from build123d import *

# Parameters (mm, degrees)
BOSS_EXTRUDE1_DEPTH = 4.51
CUT_EXTRUDE1_DEPTH  = 4.2
SKETCH6_R           = 0.65
BOSS_EXTRUDE2_DEPTH = 4.2
SKETCH7_R           = 0.55
CUT_EXTRUDE2_DEPTH  = 4.6
SKETCH8_R           = 0.5
CUT_EXTRUDE3_DEPTH  = 3.5
SKETCH10_R          = 0.5
SKETCH10_R_2        = 0.985
SKETCH10_R_3        = 0.9
SKETCH10_R_4        = 1
SKETCH10_R_5        = 0.75
CUT_EXTRUDE4_DEPTH  = 10
SKETCH16_W          = 2.4
SKETCH16_H          = 3
SKETCH16_H_2        = 1.5
CUT_EXTRUDE5_DEPTH  = 0.6
SKETCH18_W          = 1.5
SKETCH18_H          = 2.4
CUT_EXTRUDE6_DEPTH  = 1
SKETCH21_W          = 2.4
SKETCH21_H          = 1.5
SKETCH21_W_2        = 1.5
SKETCH21_H_2        = 8.25
CUT_EXTRUDE7_DEPTH  = 0.6
SKETCH22_R          = 1.3
SKETCH22_R_2        = 0.9
BOSS_EXTRUDE3_DEPTH = 4.25
SKETCH23_R          = 5.9
SKETCH23_R_2        = 5.5
BOSS_EXTRUDE4_DEPTH = 4
SKETCH24_R          = 1.6
SKETCH24_R_2        = 1.2
SKETCH24_R_3        = 1.25
SKETCH24_R_4        = 0.5
BOSS_EXTRUDE5_DEPTH = 3.75
SKETCH26_R          = 0.75
BOSS_EXTRUDE6_DEPTH = 4.51
SKETCH27_R          = 0.675
BOSS_EXTRUDE7_DEPTH = 4.6
BOSS_EXTRUDE8_DEPTH = 1.25
SKETCH29_W          = 0.2
SKETCH29_H          = 13.4
CUT_EXTRUDE8_DEPTH  = 15


with BuildPart() as part:
    # Sketch4 → Boss-Extrude1 (new body)
    with BuildSketch(Plane.XY):
        with BuildLine():
            ThreePointArc((-13.711599695, 0.852101617), (-13.847357447, 0.940933533), (-13.9, 1.09439375))
            Line((-13.9, 1.09439375), (-13.9, 24.20560625))
            ThreePointArc((-13.9, 24.20560625), (-13.847357447, 24.359066467), (-13.711599695, 24.447898383))
            Line((-13.711599695, 24.447898383), (-10.481270444, 25.269168531))
            ThreePointArc((-10.481270444, 25.269168531), (-10.359031781, 25.292262196), (-10.234871665, 25.3))
            Line((-10.234871665, 25.3), (-3.665128335, 25.3))
            ThreePointArc((-3.665128335, 25.3), (-3.540968219, 25.292262196), (-3.418729556, 25.269168531))
            Line((-3.418729556, 25.269168531), (-0.188400305, 24.447898383))
            ThreePointArc((-0.188400305, 24.447898383), (-0.052642553, 24.359066467), (0, 24.20560625))
            Line((0, 24.20560625), (0, 1.09439375))
            ThreePointArc((0, 1.09439375), (-0.052642553, 0.940933533), (-0.188400305, 0.852101617))
            Line((-0.188400305, 0.852101617), (-3.418729556, 0.030831469))
            ThreePointArc((-3.418729556, 0.030831469), (-3.540968219, 0.007737804), (-3.665128335, 0))
            Line((-3.665128335, 0), (-10.234871665, 0))
            ThreePointArc((-10.234871665, 0), (-10.359031781, 0.007737804), (-10.481270444, 0.030831469))
            Line((-10.481270444, 0.030831469), (-13.711599695, 0.852101617))
        make_face()
    extrude(amount=BOSS_EXTRUDE1_DEPTH)

    # Sketch5 → Cut-Extrude1 (cut)
    with BuildSketch(Plane(origin=(0, 0, 0), x_dir=(-1, 0, 0), z_dir=(0, 0, -1))):
        with BuildLine():
            Line((13.3, 1.366545), (13.3, 23.933455))
            Line((13.3, 23.933455), (10.333431177, 24.687667412))
            ThreePointArc((10.333431177, 24.687667412), (10.284535712, 24.696904878), (10.234871665, 24.7))
            Line((10.234871665, 24.7), (3.665128335, 24.7))
            ThreePointArc((3.665128335, 24.7), (3.615464288, 24.696904878), (3.566568823, 24.687667412))
            Line((3.566568823, 24.687667412), (0.6, 23.933455))
            Line((0.6, 23.933455), (0.6, 1.366545))
            Line((0.6, 1.366545), (3.566568823, 0.612332588))
            ThreePointArc((3.566568823, 0.612332588), (3.615464288, 0.603095122), (3.665128335, 0.6))
            Line((3.665128335, 0.6), (10.234871665, 0.6))
            ThreePointArc((10.234871665, 0.6), (10.284535712, 0.603095122), (10.333431177, 0.612332588))
            Line((10.333431177, 0.612332588), (13.3, 1.366545))
        make_face()
    extrude(amount=-CUT_EXTRUDE1_DEPTH, mode=Mode.SUBTRACT)

    # Sketch6 → Boss-Extrude2 (add)
    with BuildSketch(Plane(origin=(0, 0, 4.2), x_dir=(-1, 0, 0), z_dir=(0, 0, -1))):
        with Locations((1.112347538, 1.766545)):
            Circle(SKETCH6_R)
        with Locations((1.112347538, 23.533455)):
            Circle(SKETCH6_R)
        with Locations((1.11, 12.75)):
            Circle(SKETCH6_R)
        with Locations((12.787652462, 23.533455)):
            Circle(SKETCH6_R)
        with Locations((12.787652462, 1.766545)):
            Circle(SKETCH6_R)
        with Locations((12.79, 12.75)):
            Circle(SKETCH6_R)
    extrude(amount=BOSS_EXTRUDE2_DEPTH)

    # Sketch7 → Cut-Extrude2 (cut)
    with BuildSketch(Plane(origin=(0, 0, 0), x_dir=(-1, 0, 0), z_dir=(0, 0, -1))):
        with Locations((1.112347538, 1.766545)):
            Circle(SKETCH7_R)
        with Locations((1.11, 12.75)):
            Circle(SKETCH7_R)
        with Locations((1.112347538, 23.533455)):
            Circle(SKETCH7_R)
        with Locations(Location((12.787652462, 1.766545, 0), (0, 0, 180))):
            Circle(SKETCH7_R)
        with Locations(Location((12.787652462, 23.533455, 0), (0, 0, 180))):
            Circle(SKETCH7_R)
        with Locations(Location((12.79, 12.75, 0), (0, 0, 180))):
            Circle(SKETCH7_R)
    extrude(amount=-CUT_EXTRUDE2_DEPTH, mode=Mode.SUBTRACT)

    # Sketch8 → Cut-Extrude3 (cut)
    with BuildSketch(Plane(origin=(0, 0, 4.2), x_dir=(-1, 0, 0), z_dir=(0, 0, -1))):
        with Locations(Location((6.95, 24.2, 0), (0, 0, 90))):
            Circle(SKETCH8_R)
    extrude(amount=-CUT_EXTRUDE3_DEPTH, mode=Mode.SUBTRACT)

    # Sketch10 → Cut-Extrude4 (cut)
    with BuildSketch(Plane.XY.offset(4.51)):
        with Locations((-7.95, 19.1)):
            Circle(SKETCH10_R)
        with Locations((-3.95, 18.3)):
            Circle(SKETCH10_R_2)
        with Locations((-6.95, 13.6)):
            Circle(SKETCH10_R_3)
        with Locations((-6.95, 6.6)):
            Circle(SKETCH10_R_4)
        with Locations((-11.3, 17.35)):
            Circle(SKETCH10_R_5)
    extrude(amount=-CUT_EXTRUDE4_DEPTH, mode=Mode.SUBTRACT)

    # Sketch16 → Cut-Extrude5 (cut)
    with BuildSketch(Plane(origin=(0, 0, 0), x_dir=(0, 0, -1), z_dir=(1, 0, 0))):
        with Locations((-1.2, 16.3)):
            Rectangle(SKETCH16_W, SKETCH16_H)
        with Locations((-1.2, 11.35)):
            Rectangle(SKETCH16_W, SKETCH16_H_2)
        with Locations((-1.2, 3.25)):
            Rectangle(SKETCH16_W, SKETCH16_H_2)
    extrude(amount=-CUT_EXTRUDE5_DEPTH, mode=Mode.SUBTRACT)

    # Sketch18 → Cut-Extrude6 (cut)
    with BuildSketch(Plane(origin=(0, 0, 0), x_dir=(-1, 0, 0), z_dir=(0, -1, 0))):
        with Locations((2.95, -1.2)):
            Rectangle(SKETCH18_W, SKETCH18_H)
        with Locations((11.15, -1.2)):
            Rectangle(SKETCH18_W, SKETCH18_H)
    extrude(amount=-CUT_EXTRUDE6_DEPTH, mode=Mode.SUBTRACT)

    # Sketch21 → Cut-Extrude7 (cut)
    with BuildSketch(Plane.ZY.offset(13.9)):
        with Locations((1.2, 3.25)):
            Rectangle(SKETCH21_W, SKETCH21_H)
        with Locations((1.2, 11.35)):
            Rectangle(SKETCH21_W, SKETCH21_H)
        with Locations((0.75, 18.175)):
            Rectangle(SKETCH21_W_2, SKETCH21_H_2)
    extrude(amount=-CUT_EXTRUDE7_DEPTH, mode=Mode.SUBTRACT)

    # Sketch22 → Boss-Extrude3 (add)
    with BuildSketch(Plane(origin=(0, 0, 4.2), x_dir=(-1, 0, 0), z_dir=(0, 0, -1))):
        with Locations((6.95, 13.6)):
            Circle(SKETCH22_R)
        with Locations(Location((6.95, 13.6, 0), (0, 0, 180))):
            Circle(SKETCH22_R_2, mode=Mode.SUBTRACT)
    extrude(amount=BOSS_EXTRUDE3_DEPTH)

    # Sketch23 → Boss-Extrude4 (add)
    with BuildSketch(Plane(origin=(0, 0, 4.2), x_dir=(-1, 0, 0), z_dir=(0, 0, -1))):
        with Locations((6.95, 6.6)):
            Circle(SKETCH23_R)
        with Locations((6.95, 6.6)):
            Circle(SKETCH23_R_2, mode=Mode.SUBTRACT)
    extrude(amount=BOSS_EXTRUDE4_DEPTH)

    # Sketch24 → Boss-Extrude5 (add)
    with BuildSketch(Plane(origin=(0, 0, 4.2), x_dir=(-1, 0, 0), z_dir=(0, 0, -1))):
        with Locations((3.95, 18.3)):
            Circle(SKETCH24_R)
        with Locations((3.95, 18.3)):
            Circle(SKETCH24_R_2, mode=Mode.SUBTRACT)
        with Locations((7.95, 19.1)):
            Circle(SKETCH24_R_3)
        with Locations(Location((7.95, 19.1, 0), (0, 0, 180))):
            Circle(SKETCH24_R_4, mode=Mode.SUBTRACT)
    extrude(amount=BOSS_EXTRUDE5_DEPTH)

    # Sketch26 → Boss-Extrude6 (add)
    with BuildSketch(Plane.XY.offset(4.51)):
        with Locations((-11.3, 17.35)):
            Circle(SKETCH26_R)
    extrude(amount=-BOSS_EXTRUDE6_DEPTH)

    # Sketch27 → Boss-Extrude7 (add)
    with BuildSketch(Plane(origin=(0, 0, 0), x_dir=(-1, 0, 0), z_dir=(0, 0, -1))):
        with Locations((11.3, 17.35)):
            Circle(SKETCH27_R)
    extrude(amount=BOSS_EXTRUDE7_DEPTH)

    # Sketch28 → Boss-Extrude8 (add)
    with BuildSketch(Plane(origin=(0, 0, 0.45), x_dir=(-1, 0, 0), z_dir=(0, 0, -1))):
        with BuildLine():
            ThreePointArc((7.737135239, 20.331742097), (9.19542716, 19.206823169), (7.95, 17.85))
            ThreePointArc((7.95, 17.85), (7.865931561, 17.934068439), (7.95, 18.018136879))
            ThreePointArc((7.95, 18.018136879), (9.02656312, 19.206956355), (7.737135239, 20.160715045))
            ThreePointArc((7.737135239, 20.160715045), (7.728639485, 20.246228571), (7.737135239, 20.331742097))
        make_face()
    extrude(amount=BOSS_EXTRUDE8_DEPTH)

    # Sketch29 → Cut-Extrude8 (cut)
    with BuildSketch(Plane(origin=(0, 0, 0), x_dir=(0, 0, -1), z_dir=(1, 0, 0))):
        with Locations((-0.1, 6.7)):
            Rectangle(SKETCH29_W, SKETCH29_H)
    extrude(amount=-CUT_EXTRUDE8_DEPTH, mode=Mode.SUBTRACT)


solid = part.part
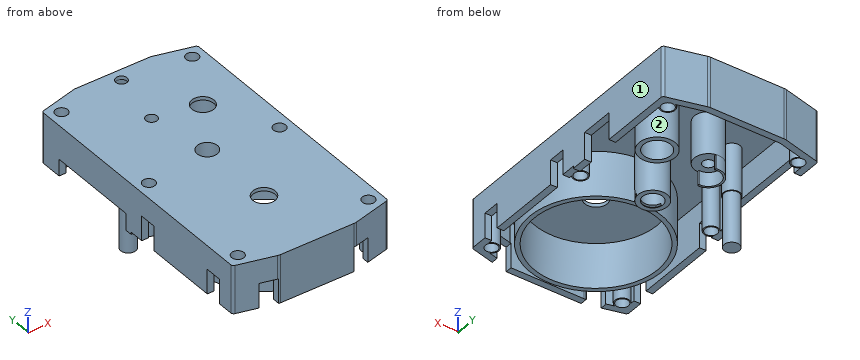
Model file for the job. Use its own axes, mm. Face numbers are marked on the shaded views. A direction names the side the tool comes from. Give positions to 0.01 mm unless a question says otherwise; leave off trailing zeros. Write each loop counter-clockwise with the first axis right and the second up, starting at its lowest first coordinate (ties: lowest second). Pieces come first, ordered by that corner, then holes. Notation, with made-up numbers: (81.5, 32.5) -> (89.5, 32.5) arc R24 ccw to (89.5, 52.5) -> close; hole circle Ø9 at (82, -37). An arc over 180 degrees is marked (long way). Write item = value, one per line.
(1) Slice it at C-C, the plane z = -1.5. Give the cut face in (x, y) (3 decimals), then the cut area to 3 significant figures.
Determined:
outline = circle Ø1.35 at (-11.3, 17.35)
area = 1.43 mm2
(2) Slice it at A-A, the plane y = 15.25. Give the cut face in (x, z).
Determined:
outline = (-13.9, 1.5) -> (-13.3, 1.5) -> (-13.3, 4.2) -> (-0.6, 4.2) -> (-0.6, 2.4) -> (0, 2.4) -> (0, 4.51) -> (-13.9, 4.51) -> close
(3) Tool access for the marked faces 1 and 2: list every direction of +Z, -Z, +X, -X, +Y, -Y with a clear straight run to the whole face (end or side of a thin tool).
Determined:
face_1 = +Z, -Z, +X, +Y, -Y
face_2 = -Z
(4) Slice it at D-D, the plane y = 5. Give the cut face in (x, z), then the cut area to 3 significant figures.
Determined:
outline = (-13.9, 0.2) -> (-13.3, 0.2) -> (-13.3, 4.2) -> (-12.63, 4.2) -> (-12.63, 0.2) -> (-12.21, 0.2) -> (-12.21, 4.2) -> (-1.69, 4.2) -> (-1.69, 0.2) -> (-1.27, 0.2) -> (-1.27, 4.2) -> (-0.6, 4.2) -> (-0.6, 0.2) -> (0, 0.2) -> (0, 4.51) -> (-13.9, 4.51) -> close
area = 12.4 mm2
(5) Flat gauge pins, fed straight in: P1, Ø3, axis at x = -6.95, y = 13.6, coming from the -Z side; P2, Ø0.7, axis at x = -0.5, z = 1.5, coming from the -Y side; P3, Ø6, axis at x = -8.5, y = 5, coming from the -Z side; P4, Ø2, axis at y = 10.5, z = -2.5, coming from the -X side (3 decimals). Where does each tip first touch, or does it go through?
Determined:
P1 = -0.05
P2 = 0.68
P3 = 4.2
P4 = through
(6) Slice it at B-B, the plane x = -3.95. Give the cut face in (y, z) (3 decimals), then the cut area to 3 significant figures.
Determined:
outline = (0, 0.2) -> (0.6, 0.2) -> (0.6, 4.2) -> (1.52, 4.2) -> (1.52, 0.2) -> (1.99, 0.2) -> (1.99, 4.2) -> (11.21, 4.2) -> (11.21, 0.2) -> (11.68, 0.2) -> (11.68, 4.2) -> (16.7, 4.2) -> (16.7, 0.45) -> (17.1, 0.45) -> (17.1, 4.2) -> (17.315, 4.2) -> (17.315, 4.51) -> (0, 4.51) -> close; (19.285, 4.2) -> (19.5, 4.2) -> (19.5, 0.45) -> (19.9, 0.45) -> (19.9, 4.2) -> (24.7, 4.2) -> (24.7, 0) -> (25.3, 0) -> (25.3, 4.51) -> (19.285, 4.51) -> close
area = 18.9 mm2
(7) Probe line 1 along Y through (x, z) = (-7.95, -0.1); line 2 along X through (y, z) = (21.5, 3.5); line 3 along X through (y, z) = (19, 3.75). List the from-to ranges inside material, lowest first.
Determined:
line_1 = 17.85 to 18.02, 20.18 to 20.35
line_2 = -13.9 to -13.3, -0.6 to 0
line_3 = -13.9 to -13.3, -9.2 to -8.44, -7.46 to -6.7, -5.39 to -4.92, -2.98 to -2.51, -0.6 to 0
